```python
from build123d import *

# Parameters (mm, degrees)
SKETCH1_R           = 7
BOSS_EXTRUDE5_DEPTH = 35
SKETCH2_R           = 10
BOSS_EXTRUDE7_DEPTH = 2
SKETCH1_19_R        = 4.05
SKETCH1_19_R_2      = 1.5
CUT_EXTRUDE2_DEPTH  = 41


with BuildPart() as part:
    # Sketch1 → Boss-Extrude5 (new body)
    with BuildSketch(Plane.XY):
        Circle(SKETCH1_R)
    extrude(amount=BOSS_EXTRUDE5_DEPTH)

    # Sketch2 → Boss-Extrude7 (add)
    with BuildSketch(Plane(origin=(0, 0, 0), x_dir=(-1, 0, 0), z_dir=(0, 0, -1))):
        Circle(SKETCH2_R)
    extrude(amount=-BOSS_EXTRUDE7_DEPTH)

    # Sketch1<19> → Cut-Extrude2 (cut)
    with BuildSketch(Plane.XY):
        Circle(SKETCH1_19_R)
        with Locations((0, 7)):
            Circle(SKETCH1_19_R_2)
        with Locations((7, 0)):
            Circle(SKETCH1_19_R_2)
        with Locations((0, -7)):
            Circle(SKETCH1_19_R_2)
        with Locations((-7, 0)):
            Circle(SKETCH1_19_R_2)
    extrude(amount=CUT_EXTRUDE2_DEPTH, mode=Mode.SUBTRACT)


solid = part.part
```
Work out the finished part from the listing and answer in its coordinate system (mm). A direction names the side the tool comes from. Coordinates: 2 decimals unless noted, no trailing zeros. Loops run counter-clockwise (first coordinate to the right, second up) from the corner with the lowest first, then second, coordinate; pieces in that order, holes last.
1) For a pull along Y with two mould halves and no side action, classify faces 4 (the flat face through (7, -2, 2)), 5 (the cylindrical face through (-0.878, -3.954, 17.255)), 6 (the cylindrical face through (-5.57, 0.45, 17.26)), 7 (the cylindrical face through (4.9, -5, 18.3)) as +Y half, -Y half, draft (parallel to the pull), parting line (faces both ways), or undercut.
Results:
face 4: draft
face 5: undercut
face 6: undercut
face 7: -Y half
2) Consider probe 1 along Y at (x, z) = (0, 18); probe 2 along X at (y, z) = (-2.5, 29.5). Determine where each line is inside the solid, lowest interval first.
Results:
probe 1: y = -5.5 to -4.05, 4.05 to 5.5
probe 2: x = -6.54 to -3.19, 3.19 to 6.54
3) For faces 1 (the cylindrical face through (5, 4.9, 18.3)), 2 (the cylindrical face through (-5, -4.9, 18.3)), 3 (the cylindrical face through (-4.9, 5, 18.3)), determine the directions among +Z, -Z, +X, -X, +Y, -Y from which every point of the face is accessible in a straight line to the end or side of a thin tool.
Results:
face 1: +Z, +X, +Y
face 2: +Z, -X, -Y
face 3: +Z, -X, +Y
4) Flat-ended cylindrical pins translate along their axes: pin 1 (1.5 mm diameter, centred on x = -6, z = 10.5, fed in from -Y); pin 2 (4 mm diameter, centred on x = 6.5, z = 20.5, fed in from +Y); pin 3 (1.5 mm diameter, centred on y = 1, z = 15.5, fed in from -X). Find the tip coordinate at first contact, or state that the pin passes through.
Results:
pin 1: stops at y = -4.63
pin 2: stops at y = 5.36
pin 3: stops at x = -6.84
5) Section B-B (z = 24) is taken. Give the vertices of the cut face in (x, y), plus the area to 3 significant figures.
Results:
outline: (-6.84, -1.49) arc R7 ccw to (-1.49, -6.84) arc R1.5 cw to (1.49, -6.84) arc R7 ccw to (6.84, -1.49) arc R1.5 cw to (6.84, 1.49) arc R7 ccw to (1.49, 6.84) arc R1.5 cw to (-1.49, 6.84) arc R7 ccw to (-6.84, 1.49) arc R1.5 cw to start; hole circle Ø8.1 at (0, 0)
area: 88.9 mm2
6) Section C-C (y = 8) is taken. Give the vertices of the cut face in (x, z).
Results:
outline: (-6, 0) - (-1.12, 0) - (-1.12, 2) - (-6, 2) - close; (1.12, 0) - (6, 0) - (6, 2) - (1.12, 2) - close
7) Section A-A (x = 0) is taken. Give the vertices of the cut face in (y, z), plus the area to 4 significant figures.
Results:
outline: (-10, 0) - (-8.5, 0) - (-8.5, 2) - (-10, 2) - close; (-5.5, 0) - (-4.05, 0) - (-4.05, 35) - (-5.5, 35) - close; (4.05, 0) - (5.5, 0) - (5.5, 35) - (4.05, 35) - close; (8.5, 0) - (10, 0) - (10, 2) - (8.5, 2) - close
area: 107.5 mm2
